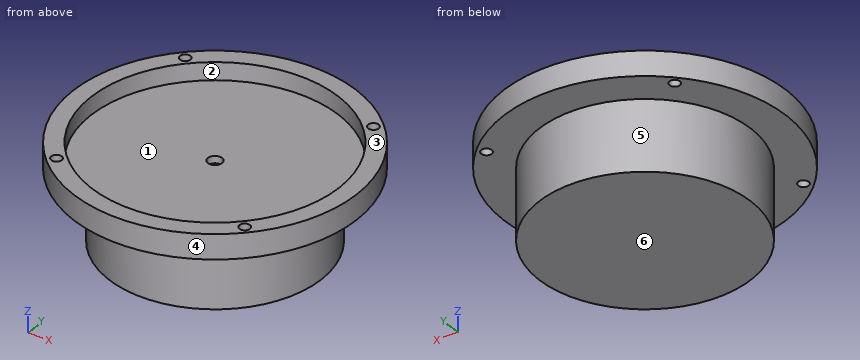
from build123d import *

# Parameters (mm, degrees)
F0_R            = 50.8
F1_DEPTH        = 2.54
F2_R            = 50.8
F2_R_2          = 44.45
F3_DEPTH        = 6.35
F5_D            = 3.7973
F5_COPIES_COUNT = 4
F7_D            = 5.1054
F8_R            = 38.1
F8_R_2          = 2.5527
F9_DEPTH        = 25.4


# Not quite as in the source:
# - a pattern or mirror of a feature is missing from the dataset's text; its kind, count and spacing are read off the source's solid


with BuildPart() as f1:
    # F0 (on Top) → F1 (new body)
    with BuildSketch(Plane.XY):
        Circle(F0_R)
    extrude(amount=F1_DEPTH)

    # F2 (on face) → F3 (join)
    with BuildSketch(Plane.XY.offset(2.54)):
        Circle(F2_R)
        Circle(F2_R_2, mode=Mode.SUBTRACT)
    extrude(amount=F3_DEPTH)

    # F5 (through all)
    with Locations(Plane.XY.offset(8.89)):
        with Locations((-33.675960454, 33.675960454)):
            f5 = Hole(F5_D / 2)

    # F5_copies: F5 ×4 about axis
    f5_copies_axis = Axis((0, 0, 0), (0, 0, 1))
    for i in range(1, F5_COPIES_COUNT):
        add(f5.rotate(f5_copies_axis, i * 360 / F5_COPIES_COUNT), mode=Mode.SUBTRACT)

    # F7 (through all)
    with Locations(Plane.XY.offset(2.54)):
        with Locations((0, 0)):
            Hole(F7_D / 2)

    # F8 (on face) → F9 (join)
    with BuildSketch(Plane(origin=(0, 0, 0), x_dir=(1, 0, 0), z_dir=(0, 0, -1))):
        Circle(F8_R)
        Circle(F8_R_2, mode=Mode.SUBTRACT)
        Circle(F8_R_2)
    extrude(amount=F9_DEPTH)


solid = f1.part
Here's how the part is built. I have some questions about the finished solid (model axes, mm). Face numbers are marked on the shaded views. A direction names the side the tool comes from. Coordinates: 2 decimals unless noted, no trailing zeros. Write each loop counter-clockwise with the first axis right and the second up, starting at its lowest first coordinate (ties: lowest second). Pieces come first, ordered by that corner, then holes.
Item 1: I want a section at A-A on x = 0. Write out the boundary of the cut face in (y, z), and give its area (3 significant figures).
Item 2: I want a section at C-C on z = 5.5. Write out the boundary of the cut face in (x, y).
Item 3: If we mould it in two halves opening along Y, with no side actions, what happens to the marked faces 1, 2, 3 and 4? For each: +Y half, -Y half, draft (parallel to the pull), parting line (faces both ways), or undercut.
Item 4: Will these pins go through, and if not, where does the flat tip stop? pin 1 (6 mm diameter, centred on y = 16.5, z = -14.5, fed in from +X); pin 2 (4 mm diameter, centred on y = 24.5, z = -9, fed in from -X); pin 3 (1.5 mm diameter, centred on x = 9.5, z = -7, fed in from -Y).
Item 5: If I drill on line 1 (Y direction, x = 0, z = 2); line 2 (Z direction, x = -9, y = 39); line 3 (Z direction, x = -39.5, y = -23), over which ranges is the centre line in solid material (lowest first)?
Item 6: On a 3-axis mill with a long thin cutter (end or side, diameter ignored), from which of +Z, -Z, +X, -X, +Y, -Y can I reach the whole of each face in a straight line? I mean the marked faces 5 and 6. Say none if no direction works.
Item 7: I want a section at D-D on z = -15. Write out the boundary of the cut face in (x, y), and give its area (3 significant figures).
Findings below:
1. outline: (-50.8, 0) - (-38.1, 0) - (-38.1, -25.4) - (38.1, -25.4) - (38.1, 0) - (50.8, 0) - (50.8, 8.89) - (44.45, 8.89) - (44.45, 2.54) - (2.55, 2.54) - (2.55, 0) - (-2.55, 0) - (-2.55, 2.54) - (-44.45, 2.54) - (-44.45, 8.89) - (-50.8, 8.89) - close
1. area: 2,260 mm2
2. outline: circle Ø101.6 at (0, 0); hole circle Ø88.9 at (0, 0); hole circle Ø3.8 at (-33.68, -33.68); hole circle Ø3.8 at (-33.68, 33.68); hole circle Ø3.8 at (33.68, -33.68); hole circle Ø3.8 at (33.68, 33.68)
3. face 1: undercut
3. face 2: undercut
3. face 3: draft
3. face 4: parting line
4. pin 1: stops at x = 35.63
4. pin 2: stops at x = -30.75
4. pin 3: stops at y = -37.08
5. line 1: y = -50.8 to -2.55, 2.55 to 50.8
5. line 2: z = 0 to 2.54
5. line 3: z = 0 to 8.89
6. face 5: -Z
6. face 6: -Z, +X, -X, +Y, -Y
7. outline: circle Ø76.2 at (0, 0)
7. area: 4,560 mm2
